Could you check a few things on this drawing? It's one solid part, dimensions in mm from its lowest x, y, z. Round coordinates to 2 decimals unless told otherwise and drop trailing zeros. Write each loop counter-clockwise with the first axis right and the second up, starting at its lowest first coordinate (ties: lowest second). Pieces come first, ordered by that corner, then holes. Notation, with made-up numbers: (65.25, 81) - (96.25, 81) arc R13 cw to (96.25, 104) - close; hole circle Ø5 at (21, 26.5). An arc over 180 degrees is marked (long way). Use one line per item in the form item = value. Start each with the question number.
1. If I drill on line 1 along Y through (x, z) = (26.5, 25); line 2 along Z through (x, y) = (43.5, 24.5); line 3 along Z through (x, y) = (12.5, 39) (1 decimal), over which ranges is the centre line in solid material (lowest first)?
2. I want a section at A-A, the plane z = 23. List the corners of the cut face in (x, y) for me.
3. I want a section at B-B, the plane y = 26.5. List the corners of the cut face in (x, z) for me, plus the area to 3 significant figures.
4. I want a section at C-C, the plane x = 31. List the corners of the cut face in (y, z) for me.
5. We'd pull the mould along Z, two halves only. Please class the marked faces 1, 2, 3 and 4: +Z half, -Z half, draft (parallel to the pull), parting line (faces both ways), or undercut.
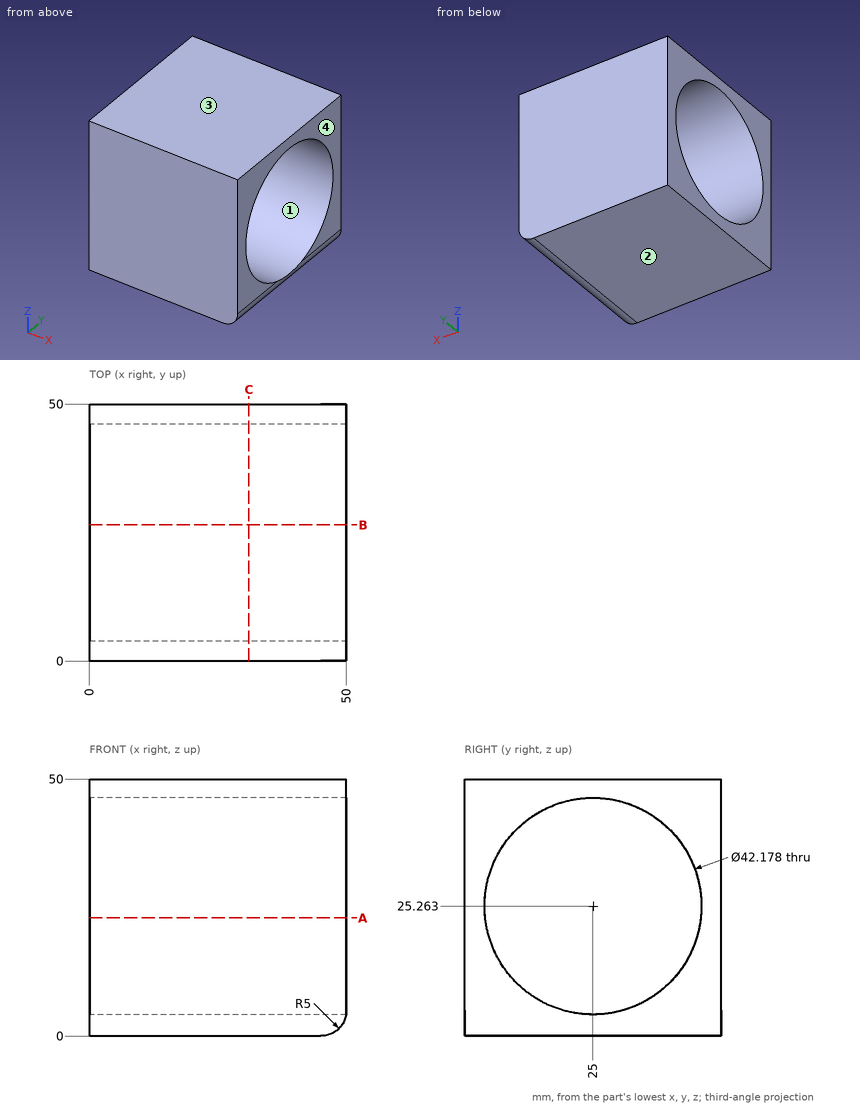
Model answer:
q1.line_1 = 0 to 3.91, 46.09 to 50
q1.line_2 = 0 to 4.18, 46.35 to 50
q1.line_3 = 0 to 9.5, 41 to 50
q2.outline = (0, 0) - (50, 0) - (50, 4.03) - (0, 4.03) - close; (0, 45.97) - (50, 45.97) - (50, 50) - (0, 50) - close
q3.outline = (0, 0) - (45, 0) arc R5 ccw to (49.94, 4.23) - (0, 4.23) - close; (0, 46.3) - (50, 46.3) - (50, 50) - (0, 50) - close
q3.area = 391 mm2
q4.outline = (0, 0) - (50, 0) - (50, 50) - (0, 50) - close; hole circle Ø42.18 at (25, 25.26)
q5.face_1 = undercut
q5.face_2 = -Z half
q5.face_3 = +Z half
q5.face_4 = draft
